```python
from build123d import *

# Parameters (mm, degrees)
SKETCH2_W        = 14.4
SKETCH2_H        = 20.6
SKETCH2_W_2      = 1
SKETCH2_H_2      = 17
TOP_DEPTH        = 3.2
SKETCH3_W        = 14.4
SKETCH3_H        = 20.6
SKETCH3_W_2      = 10.8
SKETCH3_H_2      = 17
BODY_DEPTH       = 196.8
SKETCH4_W        = 14.4
SKETCH4_H        = 20.6
SKETCH4_W_2      = 12.62
SKETCH4_H_2      = 18.82
INSERT_DEPTH     = 10
SKETCH5_W        = 0.8
SKETCH5_H        = 17
FLEX_DEPTH       = 196.8
SERVO_GEAR_REACH = 212.408
SKETCH9_R        = 2.275
CHAMFER1_SIZE    = 4


with BuildPart() as part:
    # Sketch2 → Top (new body)
    with BuildSketch(Plane.XY):
        with Locations((0.9, 0)):
            Rectangle(SKETCH2_W, SKETCH2_H)
        with Locations((5.8, 0)):
            Rectangle(SKETCH2_W_2, SKETCH2_H_2, mode=Mode.SUBTRACT)
    extrude(amount=-TOP_DEPTH)

    # Sketch3 → Body (add)
    with BuildSketch(Plane(origin=(0, 0, -3.2), x_dir=(-1, 0, 0), z_dir=(0, 0, -1))):
        with Locations((-0.9, 0)):
            Rectangle(SKETCH3_W, SKETCH3_H)
        with Locations((-0.9, 0)):
            Rectangle(SKETCH3_W_2, SKETCH3_H_2, mode=Mode.SUBTRACT)
    extrude(amount=BODY_DEPTH)

    # Sketch4 → Insert (add)
    with BuildSketch(Plane(origin=(0, 0, -200), x_dir=(-1, 0, 0), z_dir=(0, 0, -1))):
        with Locations((-0.9, 0)):
            Rectangle(SKETCH4_W, SKETCH4_H)
        with Locations((-0.9, 0)):
            Rectangle(SKETCH4_W_2, SKETCH4_H_2, mode=Mode.SUBTRACT)
    extrude(amount=INSERT_DEPTH)

    # Sketch5 → Flex (add)
    with BuildSketch(Plane(origin=(0, 0, -3.2), x_dir=(-1, 0, 0), z_dir=(0, 0, -1))):
        with Locations((-4.9, 0)):
            Rectangle(SKETCH5_W, SKETCH5_H)
    extrude(amount=FLEX_DEPTH)

    # Sketch9 → Servo gear (cut, up to next)
    with BuildSketch(Plane.XY, mode=Mode.PRIVATE) as servo_gear_sk1:
        Circle(SKETCH9_R)
    servo_gear_tool1 = extrude(servo_gear_sk1.sketch, amount=-SERVO_GEAR_REACH, mode=Mode.PRIVATE) & part.part
    add(servo_gear_tool1.solids().sort_by_distance((0, 0, 0))[0], mode=Mode.SUBTRACT)

    # Sketch15 → CSK for M2 Flat Head Machine Screw2 (revolve, cut)
    with BuildSketch(Plane(origin=(0.9, -10.3, -205), x_dir=(0, 0, -1), z_dir=(1, 0, 0))):
        Polygon((0, 0), (0, 0.89), (1.1, 0.89), (1.1, 0.85), (1.95, 0), align=None)
    revolve(axis=Axis((0.9, -16.65, -205), (0, 1, 0)), mode=Mode.SUBTRACT)

    # Sketch18 → CSK for M2 Flat Head Machine Screw3 (revolve, cut)
    with BuildSketch(Plane(origin=(0.9, 10.3, -205), x_dir=(0, 0, 1), z_dir=(1, 0, 0))):
        Polygon((0, 0), (0, 0.89), (1.1, 0.89), (1.1, 0.85), (1.95, 0), align=None)
    revolve(axis=Axis((0.9, 16.65, -205), (0, -1, 0)), mode=Mode.SUBTRACT)

    # Chamfer1
    chamfer1_edges = [part.edges().sort_by_distance(p)[0] for p in [
        (-4.5, -8.5, -101.6),
        (-4.5, 8.5, -101.6),
        (4.5, 8.5, -101.6),
        (4.5, -8.5, -101.6),
    ]]
    chamfer(chamfer1_edges, length=CHAMFER1_SIZE)


solid = part.part
```
Geometry check sheet. Reference: the model listing, model coordinates, mm. A direction names the side the tool comes from. Give positions to 0.01 mm unless a question says otherwise; leave off trailing zeros. Write each loop counter-clockwise with the first axis right and the second up, starting at its lowest first coordinate (ties: lowest second). Pieces come first, ordered by that corner, then holes. Notation, with made-up numbers: (82, 0.25) - (127, 0.25) arc R11 cw to (127, 15.25) - close; hole circle Ø5 at (17, -28.75). An arc over 180 degrees is marked (long way). Use a Markdown table: item, result.
Q1. Set-up check for faces 4 (the face through (5.3, 0, -99)), 5 (the face through (2.4, -9.41, -204.9)), 6 (the face through (8.1, 0, -104)): record each of +Z, -Z, +X, -X, +Y, -Y from which the full face is reachable in a straight line by a thin tool's end or side.
Computed:
| item | result |
|---|---|
| face 4 | +Z, -Z |
| face 5 | -Z |
| face 6 | +Z, -Z, +X, +Y, -Y |
Q2. Go/stop test with flat-tipped pins: P1, Ø4, axis at x = -0.5, y = 3, coming from the -Z side; P2, Ø3, axis at x = 4.5, y = 8, coming from the +Z side. Record where each tip stops, or that it passes through.
Computed:
| item | result |
|---|---|
| P1 | stops at z = -3.2 |
| P2 | stops at z = 0 |
Q3. Section check B-B, the plane z = -131.5. Enter the section's corners in (x, y).
Computed:
| item | result |
|---|---|
| outline | (-6.3, -10.3) - (8.1, -10.3) - (8.1, 10.3) - (-6.3, 10.3) - close; hole (-4.5, -4.5) - (-0.5, -8.5) - (0.5, -8.5) - (4.5, -4.5) - (4.5, 4.5) - (0.5, 8.5) - (-0.5, 8.5) - (-4.5, 4.5) - close; hole (5.3, -8.5) - (6.3, -8.5) - (6.3, 8.5) - (5.3, 8.5) - close |
Q4. Section check A-A, the plane y = 0. Enter the section's corners in (x, z) (3 decimals), then the cut area to 3 significant figures.
Computed:
| item | result |
|---|---|
| outline | (-6.3, -210) - (-5.41, -210) - (-5.41, -200) - (-4.5, -200) - (-4.5, -3.2) - (-2.275, -3.2) - (-2.275, 0) - (-6.3, 0) - close; (2.275, -3.2) - (4.5, -3.2) - (4.5, -200) - (5.3, -200) - (5.3, 0) - (2.275, 0) - close; (6.3, -200) - (7.21, -200) - (7.21, -210) - (8.1, -210) - (8.1, 0) - (6.3, 0) - close |
| area | 912 mm² |
Q5. Draft check along Y on faces 1 (the face through (0.8, 2.4, 0)), 2 (the face through (1, -10.3, -104)), 3 (the face through (2, 7, -100)). Enter one of: pulls with the +Y half, pulls with the -Y half, needs draft (parallel to the pull), parting line crosses it, or undercut.
Computed:
| item | result |
|---|---|
| face 1 | needs draft |
| face 2 | pulls with the -Y half |
| face 3 | undercut |
Q6. Thickness scan on L1, parallel to X at y = -2, z = -112.5; L2, parallel to Y at x = -0.5, z = -173; L3, parallel to X at y = -5.75, z = -126. Record the ranges inside material, lowest first. Write a range as [from, to].
Computed:
| item | result |
|---|---|
| L1 | x = [-6.3, -4.5], [4.5, 5.3], [6.3, 8.1] |
| L2 | y = [-10.3, -8.5], [8.5, 10.3] |
| L3 | x = [-6.3, -3.25], [3.25, 5.3], [6.3, 8.1] |
